Here's how the part is built. I have some questions about the finished solid (model axes, mm). Face numbers are marked on the shaded views. A direction names the side the tool comes from. Coordinates: 2 decimals unless noted, no trailing zeros. Loops run counter-clockwise (first coordinate to the right, second up) from the corner with the lowest first, then second, coordinate; pieces in that order, holes last.
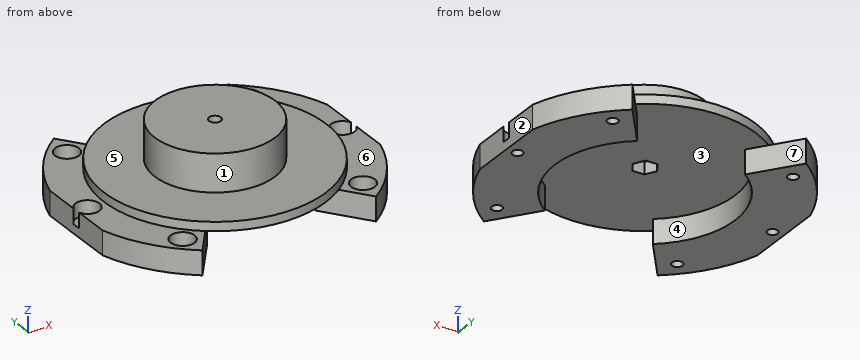
from build123d import *

# Parameters (mm, degrees)
SKETCH1_R           = 48.25
BOSS_EXTRUDE1_DEPTH = 8
SKETCH2_W           = 17.162038191
SKETCH2_H           = 56.822210482
SKETCH2_W_2         = 16.152506533
SKETCH2_H_2         = 65.186901365
CUT_EXTRUDE1_DEPTH  = 8
SKETCH3_R           = 30
CUT_EXTRUDE2_DEPTH  = 8
SKETCH4_R           = 1.75
CUT_EXTRUDE3_DEPTH  = 10
CIRPATTERN1_COUNT   = 8
CUT_EXTRUDE4_DEPTH  = 10
CIRPATTERN2_COUNT   = 2
SKETCH9_R           = 4
CUT_EXTRUDE5_DEPTH  = 5
CIRPATTERN3_COUNT   = 8
SKETCH10_R          = 4
CUT_EXTRUDE6_DEPTH  = 5
SKETCH11_R          = 37
BOSS_EXTRUDE2_DEPTH = 3
SKETCH12_R          = 20
BOSS_EXTRUDE3_DEPTH = 12.5
SKETCH13_R          = 2
CUT_EXTRUDE8_DEPTH  = 38
CUT_EXTRUDE9_DEPTH  = 4


with BuildPart() as part:
    # Sketch1 → Boss-Extrude1 (new body)
    with BuildSketch(Plane.XY):
        Circle(SKETCH1_R)
    extrude(amount=-BOSS_EXTRUDE1_DEPTH)

    # Sketch2 → Cut-Extrude1 (cut)
    with BuildSketch(Plane.XY):
        with Locations((-54.831019095, 0)):
            Rectangle(SKETCH2_W, SKETCH2_H)
        with Locations((54.326253267, -4.182345442)):
            Rectangle(SKETCH2_W_2, SKETCH2_H_2)
    extrude(amount=-CUT_EXTRUDE1_DEPTH, mode=Mode.SUBTRACT)

    # Sketch3 → Cut-Extrude2 (cut)
    with BuildSketch(Plane.XY):
        Circle(SKETCH3_R)
    extrude(amount=-CUT_EXTRUDE2_DEPTH, mode=Mode.SUBTRACT)

    # Sketch4 → Cut-Extrude3 (cut)
    with BuildSketch(Plane.XY):
        with Locations((-42.5, 0)):
            Circle(SKETCH4_R)
    cut_extrude3 = extrude(amount=-CUT_EXTRUDE3_DEPTH, mode=Mode.SUBTRACT)

    # CirPattern1: Cut-Extrude3 ×8 about axis
    cirpattern1_axis = Axis((0, 0, 0), (0, 0, 1))
    for i in range(1, CIRPATTERN1_COUNT):
        add(cut_extrude3.rotate(cirpattern1_axis, i * 360 / CIRPATTERN1_COUNT), mode=Mode.SUBTRACT)

    # Sketch8 → Cut-Extrude4 (cut)
    with BuildSketch(Plane.XY):
        with BuildLine():
            Line((-28.959547499, 38.59283753), (0, 0))
            Line((0, 0), (28.959547499, 38.59283753))
            ThreePointArc((28.959547499, 38.59283753), (0, 48.25), (-28.959547499, 38.59283753))
        make_face()
    cut_extrude4 = extrude(amount=-CUT_EXTRUDE4_DEPTH, mode=Mode.SUBTRACT)

    # CirPattern2: Cut-Extrude4 ×2 about axis
    cirpattern2_axis = Axis((0, 0, 0), (0, 0, 1))
    for i in range(1, CIRPATTERN2_COUNT):
        add(cut_extrude4.rotate(cirpattern2_axis, i * 360 / CIRPATTERN2_COUNT), mode=Mode.SUBTRACT)

    # Sketch9 → Cut-Extrude5 (cut)
    with BuildSketch(Plane.XY):
        with Locations((-42.5, 0)):
            Circle(SKETCH9_R)
    cut_extrude5 = extrude(amount=-CUT_EXTRUDE5_DEPTH, mode=Mode.SUBTRACT)

    # CirPattern3: Cut-Extrude5 ×8 about axis, 3 skipped
    cirpattern3_axis = Axis((0, 0, 0), (0, 0, 1))
    add([cut_extrude5.rotate(cirpattern3_axis, i * 360 / CIRPATTERN3_COUNT) for i in range(1, CIRPATTERN3_COUNT) if i not in (3, 4, 5)], mode=Mode.SUBTRACT)

    # Sketch10 → Cut-Extrude6 (cut)
    with BuildSketch(Plane.XY):
        with Locations((42.5, 0)):
            Circle(SKETCH10_R)
        with Locations((30.0520382, 30.0520382)):
            Circle(SKETCH10_R)
        with Locations((30.0520382, -30.0520382)):
            Circle(SKETCH10_R)
    extrude(amount=-CUT_EXTRUDE6_DEPTH, mode=Mode.SUBTRACT)

    # Sketch11 → Boss-Extrude2 (add)
    with BuildSketch(Plane.XY):
        with Locations(Location((0, 0, 0), (0, 0, 126.884070759))):
            Circle(SKETCH11_R)
    extrude(amount=BOSS_EXTRUDE2_DEPTH)

    # Sketch12 → Boss-Extrude3 (add)
    with BuildSketch(Plane.XY.offset(3)):
        Circle(SKETCH12_R)
    extrude(amount=BOSS_EXTRUDE3_DEPTH)

    # Sketch13 → Cut-Extrude8 (cut)
    with BuildSketch(Plane.XY.offset(15.5)):
        Circle(SKETCH13_R)
    extrude(amount=-CUT_EXTRUDE8_DEPTH, mode=Mode.SUBTRACT)

    # Sketch14 → Cut-Extrude9 (cut)
    with BuildSketch(Plane(origin=(0, 0, 0), x_dir=(-1, 0, 0), z_dir=(0, 0, -1))):
        Polygon((-2.020725942, -3.5), (2.020725942, -3.5), (4.041451884, 0), (2.020725942, 3.5), (-2.020725942, 3.5), (-4.041451884, 0), align=None)
    extrude(amount=-CUT_EXTRUDE9_DEPTH, mode=Mode.SUBTRACT)


solid = part.part
Q1. We'd pull the mould along X, two halves only. Please class the marked faces 1, 2 and 3: pulls with the +X half, pulls with the -X half, needs draft (parallel to the pull), parting line crosses it, or undercut.
Q2. Suppose I cut it at A-A on x = 0. Write out the boundary of the cut face in (y, z).
Q3. Suppose I cut it at C-C on z = 13.75. Write out the boundary of the cut face in (x, y).
Q4. Will these pins go through, and if not, where does the flat tip stop? P1, Ø7, axis at x = 42.5, y = 0, coming from the -Z side; P2, Ø3, axis at x = 30.05, y = 30.05, coming from the +Z side; P3, Ø8.5, axis at x = 42, y = -1, coming from the +Z side; P4, Ø2, axis at x = 1.5, y = 1, coming from the -Z side.
Q5. Suppose I cut it at D-D on y = 7. Write out the boundary of the cut face in (x, z) (3 decimals).
Q6. Please list where these lines run through material, in increasing order: probe 1 along Y at (x, z) = (31, -5.5); probe 2 along Z at (x, y) = (-9, -11); probe 3 along Z at (x, y) = (29, -23.5).
Q7. For the marked faces 4, 5, 6 and 7, which set-ups out of +Z, -Z, +X, -X, +Y, -Y let a thin tool reach every point of the face, with its end or its side?
Q8. Suppose I cut it at B-B on z = -2.5. Write out the boundary of the cut face in (x, y).
Check values:
1. face 1: parting line crosses it
1. face 2: pulls with the +X half
1. face 3: undercut
2. outline: (-37, 0) - (-3.5, 0) - (-3.5, 4) - (-2, 4) - (-2, 15.5) - (-20, 15.5) - (-20, 3) - (-37, 3) - close; (2, 4) - (3.5, 4) - (3.5, 0) - (37, 0) - (37, 3) - (20, 3) - (20, 15.5) - (2, 15.5) - close
3. outline: circle Ø40 at (0, 0); hole circle Ø4 at (0, 0)
4. P1: stops at z = -8
4. P2: passes through
4. P3: stops at z = 0
4. P4: stops at z = 4
5. outline: (-46.25, -8) - (-29.172, -8) - (-29.172, 0) - (29.172, 0) - (29.172, -8) - (46.25, -8) - (46.25, 0) - (36.332, 0) - (36.332, 3) - (18.735, 3) - (18.735, 15.5) - (-18.735, 15.5) - (-18.735, 3) - (-36.332, 3) - (-36.332, 0) - (-46.25, 0) - close
6. probe 1: y = -36.97 to -31.52, -28.58 to 28.58, 31.52 to 36.97
6. probe 2: z = 0 to 15.5
6. probe 3: z = -8 to 0
7. face 4: -Z
7. face 5: +Z
7. face 6: +Z, +X
7. face 7: -Z, +Y
8. outline: (-46.25, -13.75) arc R48.25 ccw to (-28.96, -38.59) - (-18.01, -24) arc R30 cw to (-18.01, 24) - (-28.96, 38.59) arc R48.25 ccw to (-46.25, 13.75) - (-46.25, 1.39) arc R4 cw (long way) to (-46.25, -1.39) - close; (18.01, -24) - (28.96, -38.59) arc R48.25 ccw to (46.25, -13.75) - (46.25, -1.39) arc R4 cw (long way) to (46.25, 1.39) - (46.25, 13.75) arc R48.25 ccw to (28.96, 38.59) - (18.01, 24) arc R30 cw to start; hole circle Ø8 at (-30.05, -30.05); hole circle Ø8 at (-30.05, 30.05); hole circle Ø8 at (30.05, -30.05); hole circle Ø8 at (30.05, 30.05)
